```python
from build123d import *

# Parameters (mm, degrees)
SKETCH1_R           = 40
BOSS_EXTRUDE1_DEPTH = 30
SKETCH2_R           = 35
CUT_EXTRUDE1_DEPTH  = 25
CUT_EXTRUDE2_REACH  = 66.031
SKETCH4_R           = 6
SKETCH4_R_2         = 1


with BuildPart() as part:
    # Sketch1 → Boss-Extrude1 (new body)
    with BuildSketch(Plane(origin=(0, 0, 0), x_dir=(1, 0, 0), z_dir=(0, 1, 0))):
        with Locations(Location((0, 0, 0), (0, 0, 270))):
            Circle(SKETCH1_R)
    extrude(amount=BOSS_EXTRUDE1_DEPTH)

    # Sketch2 → Cut-Extrude1 (cut)
    with BuildSketch(Plane(origin=(0, 30, 0), x_dir=(1, 0, 0), z_dir=(0, 1, 0))):
        with Locations(Location((0, 0, 0), (0, 0, 270))):
            Circle(SKETCH2_R)
    extrude(amount=-CUT_EXTRUDE1_DEPTH, mode=Mode.SUBTRACT)

    # Sketch4 → Cut-Extrude2 (cut, up to next)
    with BuildSketch(Plane.XZ, mode=Mode.PRIVATE) as cut_extrude2_sk1:
        with Locations(Location((0, 0, 0), (0, 0, 270))):
            Circle(SKETCH4_R)
    cut_extrude2_tool1 = extrude(cut_extrude2_sk1.sketch, amount=-CUT_EXTRUDE2_REACH, mode=Mode.PRIVATE) & part.part
    # Sketch4 → Cut-Extrude2 (cut, up to next)
    with BuildSketch(Plane.XZ, mode=Mode.PRIVATE) as cut_extrude2_sk2:
        with Locations(Location((0, 16.383, 0), (0, 0, 270))):
            Circle(SKETCH4_R_2)
    cut_extrude2_tool2 = extrude(cut_extrude2_sk2.sketch, amount=-CUT_EXTRUDE2_REACH, mode=Mode.PRIVATE) & part.part
    # Sketch4 → Cut-Extrude2 (cut, up to next)
    with BuildSketch(Plane.XZ, mode=Mode.PRIVATE) as cut_extrude2_sk3:
        with Locations(Location((-16.383, 0, 0), (0, 0, 270))):
            Circle(SKETCH4_R_2)
    cut_extrude2_tool3 = extrude(cut_extrude2_sk3.sketch, amount=-CUT_EXTRUDE2_REACH, mode=Mode.PRIVATE) & part.part
    # Sketch4 → Cut-Extrude2 (cut, up to next)
    with BuildSketch(Plane.XZ, mode=Mode.PRIVATE) as cut_extrude2_sk4:
        with Locations(Location((16.383, 0, 0), (0, 0, 270))):
            Circle(SKETCH4_R_2)
    cut_extrude2_tool4 = extrude(cut_extrude2_sk4.sketch, amount=-CUT_EXTRUDE2_REACH, mode=Mode.PRIVATE) & part.part
    # Sketch4 → Cut-Extrude2 (cut, up to next)
    with BuildSketch(Plane.XZ, mode=Mode.PRIVATE) as cut_extrude2_sk5:
        with Locations(Location((0, -16.383, 0), (0, 0, 270))):
            Circle(SKETCH4_R_2)
    cut_extrude2_tool5 = extrude(cut_extrude2_sk5.sketch, amount=-CUT_EXTRUDE2_REACH, mode=Mode.PRIVATE) & part.part
    # Sketch4 → Cut-Extrude2 (cut, up to next)
    with BuildSketch(Plane.XZ, mode=Mode.PRIVATE) as cut_extrude2_sk6:
        with BuildLine():
            ThreePointArc((-1.496156575, 32.793473919), (-13.931787596, 29.72466502), (-24.246430247, 22.130545327))
            ThreePointArc((-24.246430247, 22.130545327), (-23.9352707, 15.31040186), (-17.115127233, 15.621561407))
            ThreePointArc((-17.115127233, 15.621561407), (-9.834203009, 20.982116485), (-1.056110524, 23.148334531))
            ThreePointArc((-1.056110524, 23.148334531), (3.546436145, 28.190927251), (-1.496156575, 32.793473919))
        make_face()
    cut_extrude2_tool6 = extrude(cut_extrude2_sk6.sketch, amount=-CUT_EXTRUDE2_REACH, mode=Mode.PRIVATE) & part.part
    # Sketch4 → Cut-Extrude2 (cut, up to next)
    with BuildSketch(Plane.XZ, mode=Mode.PRIVATE) as cut_extrude2_sk7:
        with BuildLine():
            ThreePointArc((32.793473919, 1.496156575), (29.72466502, 13.931787596), (22.130545327, 24.246430247))
            ThreePointArc((22.130545327, 24.246430247), (15.31040186, 23.9352707), (15.621561407, 17.115127233))
            ThreePointArc((15.621561407, 17.115127233), (20.982116485, 9.834203009), (23.148334531, 1.056110524))
            ThreePointArc((23.148334531, 1.056110524), (28.190927251, -3.546436145), (32.793473919, 1.496156575))
        make_face()
    cut_extrude2_tool7 = extrude(cut_extrude2_sk7.sketch, amount=-CUT_EXTRUDE2_REACH, mode=Mode.PRIVATE) & part.part
    # Sketch4 → Cut-Extrude2 (cut, up to next)
    with BuildSketch(Plane.XZ, mode=Mode.PRIVATE) as cut_extrude2_sk8:
        with BuildLine():
            ThreePointArc((1.496156575, -32.793473919), (13.931787596, -29.72466502), (24.246430247, -22.130545327))
            ThreePointArc((24.246430247, -22.130545327), (23.9352707, -15.31040186), (17.115127233, -15.621561407))
            ThreePointArc((17.115127233, -15.621561407), (9.834203009, -20.982116485), (1.056110524, -23.148334531))
            ThreePointArc((1.056110524, -23.148334531), (-3.546436145, -28.190927251), (1.496156575, -32.793473919))
        make_face()
    cut_extrude2_tool8 = extrude(cut_extrude2_sk8.sketch, amount=-CUT_EXTRUDE2_REACH, mode=Mode.PRIVATE) & part.part
    # Sketch4 → Cut-Extrude2 (cut, up to next)
    with BuildSketch(Plane.XZ, mode=Mode.PRIVATE) as cut_extrude2_sk9:
        with BuildLine():
            ThreePointArc((-32.793473919, -1.496156575), (-29.72466502, -13.931787596), (-22.130545327, -24.246430247))
            ThreePointArc((-22.130545327, -24.246430247), (-15.31040186, -23.9352707), (-15.621561407, -17.115127233))
            ThreePointArc((-15.621561407, -17.115127233), (-20.982116485, -9.834203009), (-23.148334531, -1.056110524))
            ThreePointArc((-23.148334531, -1.056110524), (-28.190927251, 3.546436145), (-32.793473919, -1.496156575))
        make_face()
    cut_extrude2_tool9 = extrude(cut_extrude2_sk9.sketch, amount=-CUT_EXTRUDE2_REACH, mode=Mode.PRIVATE) & part.part
    add(cut_extrude2_tool1.solids().sort_by_distance((0, 0, 0))[0], mode=Mode.SUBTRACT)
    add(cut_extrude2_tool2.solids().sort_by_distance((0, 0, 16.383))[0], mode=Mode.SUBTRACT)
    add(cut_extrude2_tool3.solids().sort_by_distance((-16.383, 0, 0))[0], mode=Mode.SUBTRACT)
    add(cut_extrude2_tool4.solids().sort_by_distance((16.383, 0, 0))[0], mode=Mode.SUBTRACT)
    add(cut_extrude2_tool5.solids().sort_by_distance((0, 0, -16.383))[0], mode=Mode.SUBTRACT)
    add(cut_extrude2_tool6.solids().sort_by_distance((-11.425701, 0, 24.377715))[0], mode=Mode.SUBTRACT)
    add(cut_extrude2_tool7.solids().sort_by_distance((24.377715, 0, 11.425701))[0], mode=Mode.SUBTRACT)
    add(cut_extrude2_tool8.solids().sort_by_distance((11.425701, 0, -24.377715))[0], mode=Mode.SUBTRACT)
    add(cut_extrude2_tool9.solids().sort_by_distance((-24.377715, 0, -11.425701))[0], mode=Mode.SUBTRACT)


solid = part.part
```
Verification items for the finished model (mm, model axes). A direction names the side the tool comes from. Round coordinates to 2 decimals unless told otherwise and drop trailing zeros. Write each loop counter-clockwise with the first axis right and the second up, starting at its lowest first coordinate (ties: lowest second). Pieces come first, ordered by that corner, then holes. Notation, with made-up numbers: (29.25, -21.5) -> (76.25, -21.5) arc R15 ccw to (76.25, -4.5) -> close; hole circle Ø6 at (-16.5, 87). An arc over 180 degrees is marked (long way). Write each question's results on one line, items separated by ' | '.
Q1. Sectioned sample at B-B, the plane z = 0. Record the boundary of the cut face in (x, y).
Derived:
outline: (-40, 0) -> (-32.63, 0) -> (-32.63, 5) -> (-35, 5) -> (-35, 30) -> (-40, 30) -> close; (-23.32, 0) -> (-17.38, 0) -> (-17.38, 5) -> (-23.32, 5) -> close; (-15.38, 0) -> (-6, 0) -> (-6, 5) -> (-15.38, 5) -> close; (6, 0) -> (15.38, 0) -> (15.38, 5) -> (6, 5) -> close; (17.38, 0) -> (23.32, 0) -> (23.32, 5) -> (17.38, 5) -> close; (32.63, 0) -> (40, 0) -> (40, 30) -> (35, 30) -> (35, 5) -> (32.63, 5) -> close
Q2. Draft check along Z on faces 4 (the face through (15.407, 2.465, 0.217)), 5 (the face through (29.8, 2.46, 13.77)), 6 (the face through (-8, 0, -1)), 7 (the face through (-39.05, 14.79, -8.67)). Enter one of: released by +Z, released by -Z, zero draft, split by the parting line, or undercut.
Derived:
face 4: undercut | face 5: undercut | face 6: zero draft | face 7: split by the parting line
Q3. Go/stop test with flat-tipped pins: pin 1 Ø10 at (x, z) = (20, 10) entering from +Y; pin 2 Ø4 at (y, z) = (17.5, -30.5) entering from +X; pin 3 Ø10 at (y, z) = (10, -16.5) entering from -X. Record where each tip stops, or that it passes through.
Derived:
pin 1: stops at y = 5 | pin 2: stops at x = 28.07 | pin 3: stops at x = -38.31
Q4. Thickness scan on probe 1 along X at (y, z) = (3.65, 0); probe 2 along X at (y, z) = (15, -2); probe 3 along X at (y, z) = (10, -21.5). Record the ranges inside material, lowest first.
Derived:
probe 1: x = -40 to -32.63, -23.32 to -17.38, -15.38 to -6, 6 to 15.38, 17.38 to 23.32, 32.63 to 40 | probe 2: x = -39.95 to -34.94, 34.94 to 39.95 | probe 3: x = -33.73 to -27.62, 27.62 to 33.73
Q5. Sectioned sample at A-A, the plane x = -28. Record the boundary of the cut face in (y, z).
Derived:
outline: (0, -28.57) -> (30, -28.57) -> (30, -21) -> (5, -21) -> (5, -17.14) -> (0, -17.14) -> close; (0, 3.55) -> (5, 3.55) -> (5, 21) -> (30, 21) -> (30, 28.57) -> (0, 28.57) -> close
Q6. Access from +Z, -Z, +X, -X, +Y, -Y to the whole of each face (thin tool, end or side, straight path). Record for faces 1 (the face through (13.77, 2.46, -29.8)), 2 (the face through (-7, 5, 0)), 3 (the face through (-35.4, 30, -0.2)).
Derived:
face 1: +Y, -Y | face 2: +Y | face 3: +Z, -Z, +X, -X, +Y
Q7. Sectioned sample at D-D, the plane y = 6.75. Record the boundary of the cut face in (x, z).
Derived:
outline: circle Ø80 at (0, 0); hole circle Ø70 at (0, 0)
Q8. Sectioned sample at C-C, the plane z = -29.5. Record the boundary of the cut face in (x, y).
Derived:
outline: (-27.01, 0) -> (-3.3, 0) -> (-3.3, 5) -> (-18.83, 5) -> (-18.83, 30) -> (-27.01, 30) -> close; (14.4, 0) -> (27.01, 0) -> (27.01, 30) -> (18.83, 30) -> (18.83, 5) -> (14.4, 5) -> close
